Geometry check sheet. Reference: drawing and pictorial views, mm from the part's lowest x, y, z. Round coordinates to 2 decimals unless told otherwise and drop trailing zeros. Write each loop counter-clockwise with the first axis right and the second up, starting at its lowest first coordinate (ties: lowest second). Pieces come first, ordered by that corner, then holes. Notation, with made-up numbers: (-1.75, -38) - (14.25, -38) arc R20 cw to (14.25, -26) - close; hole circle Ø4 at (74.5, 43). An arc over 180 degrees is marked (long way). Return JSON: item names as keys, results as strings.
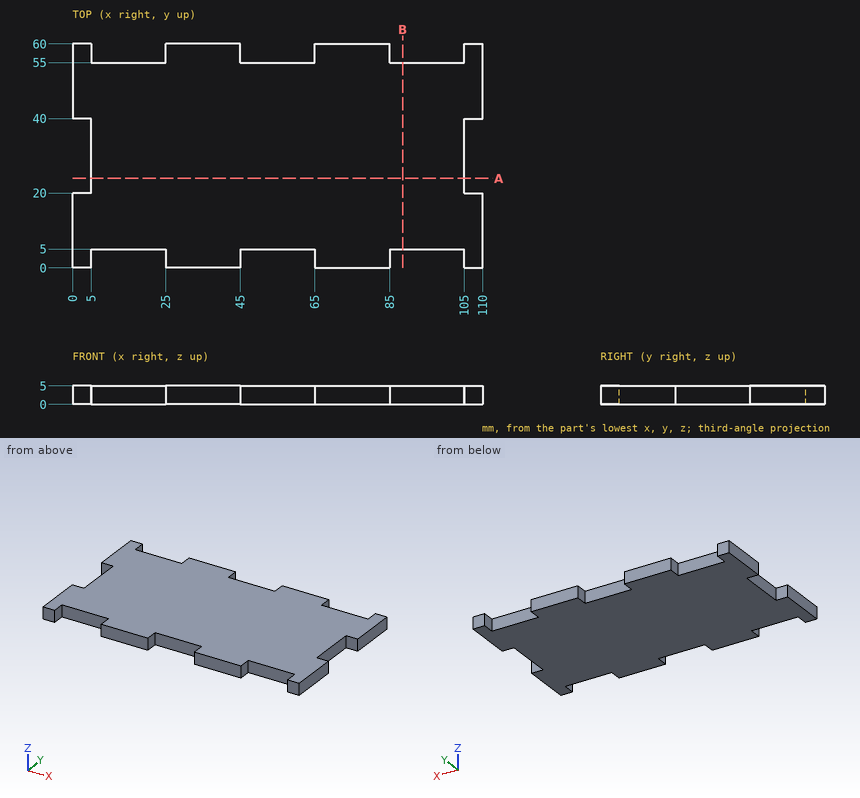
(1) Section check B-B, the plane x = 88.5. Enter the section's corners in (y, z).
Response values:
{"outline": "(5, 0) - (55, 0) - (55, 5) - (5, 5) - close"}
(2) Section check A-A, the plane y = 24. Enter the section's corners in (x, z), plus the area to 3 significant figures.
Response values:
{"outline": "(5, 0) - (105, 0) - (105, 5) - (5, 5) - close", "area": "500 mm^2"}
(3) Material ranges on line 1 along X through (y, z) = (37, 3.95); line 2 along Y through (x, z) = (92, 1.95), recorded low to high. Write a range as [from, to].
Response values:
{"line 1": "x = [5, 105]", "line 2": "y = [5, 55]"}
(4) Gauge pin test, flat ends, axial feed: pin 1 (1.5 mm diameter, centred on x = 16, z = 2, fed in from -Y); pin 2 (1.5 mm diameter, centred on y = 58.5, z = 2.5, fed in from -X). Record the tip position at first contact, or that the pin passes through.
Response values:
{"pin 1": "stops at y = 5", "pin 2": "stops at x = 0"}
